```python
from build123d import *

# Parameters (mm, degrees)
SKETCH006_R             = 1.75
SKETCH006_W             = 6.5
SKETCH006_H             = 3
SKETCH006_W_2           = 11.5
PAD001_DEPTH            = 8.5
FILLET004_R             = 1
FILLET005_R             = 0.8
FILLET006_R             = 0.5
SKETCH007_W             = 25.7
SKETCH007_H             = 13
POCKET002_DEPTH         = 3
FILLET007_R             = 0.5
SKETCH008_R             = 1.8
POCKET003_DEPTH         = 2
BODY001_PLACEMENT_ANGLE = 180


with BuildPart() as part:
    # Sketch006 → Pad001 (new body)
    with BuildSketch(Plane.XZ):
        with BuildLine():
            Line((15.7, 8.35), (15.7, -0.06))
            Line((15.7, -0.06), (16.99, -0.06))
            ThreePointArc((18.99, -2.06), (18.404214, -0.645786), (16.99, -0.06))
            Line((18.99, -2.06), (18.99, -5.56))
            ThreePointArc((16.99, -7.56), (18.404214, -6.974214), (18.99, -5.56))
            Line((16.99, -7.56), (15.7, -7.56))
            Line((15.7, -8.35), (15.7, -7.56))
            ThreePointArc((14.7, -9.35), (15.407107, -9.057107), (15.7, -8.35))
            Line((14.7, -9.35), (12, -9.35))
            Line((12, -7.41), (12, -9.35))
            Line((-12, -7.41), (12, -7.41))
            Line((-12, -7.41), (-12, -9.35))
            Line((-12, -9.35), (-13.7, -9.35))
            ThreePointArc((-14.7, -8.35), (-14.407107, -9.057107), (-13.7, -9.35))
            Line((-14.7, -8.35), (-14.7, 10.64))
            ThreePointArc((-12.7, 12.64), (-14.114214, 12.054214), (-14.7, 10.64))
            Line((-12.7, 12.64), (-8.41, 12.64))
            ThreePointArc((-6.41, 10.64), (-6.995786, 12.054214), (-8.41, 12.64))
            Line((-6.41, 10.64), (-6.41, 9.35))
            Line((-6.41, 9.35), (14.7, 9.35))
            ThreePointArc((15.7, 8.35), (15.407107, 9.057107), (14.7, 9.35))
        make_face()
        with Locations((-10.16, 8.89)):
            Circle(SKETCH006_R, mode=Mode.SUBTRACT)
        with Locations((15.24, -3.81)):
            Circle(SKETCH006_R, mode=Mode.SUBTRACT)
        with Locations((-8.91, -3.81)):
            Rectangle(SKETCH006_W, SKETCH006_H, mode=Mode.SUBTRACT)
        with Locations((6.41, -3.81)):
            Rectangle(SKETCH006_W_2, SKETCH006_H, mode=Mode.SUBTRACT)
    extrude(amount=-PAD001_DEPTH)

    # Fillet004
    fillet004_edges = [part.edges().sort_by_distance(p)[0] for p in [
        (12.16, 4.25, -2.31),
        (0.66, 4.25, -2.31),
        (-12.16, 4.25, -2.31),
        (-5.66, 4.25, -2.31),
        (12.16, 4.25, -5.31),
        (-5.66, 4.25, -5.31),
        (-12.16, 4.25, -5.31),
        (0.66, 4.25, -5.31),
    ]]
    fillet(fillet004_edges, radius=FILLET004_R)

    # Fillet005
    fillet005_edges = [part.edges().sort_by_distance(p)[0] for p in [
        (15.7, 4.25, -7.56),
        (15.7, 4.25, -0.06),
        (-6.41, 4.25, 9.35),
        (12, 4.25, -9.35),
        (-12, 4.25, -9.35),
    ]]
    fillet(fillet005_edges, radius=FILLET005_R)

    # Fillet006
    fillet006_edges = [part.edges().sort_by_distance(p)[0] for p in [
        (-12, 4.25, -7.41),
        (12, 4.25, -7.41),
    ]]
    fillet(fillet006_edges, radius=FILLET006_R)

    # Sketch007 (on Face47 of Fillet006) → Pocket002 (cut)
    with BuildSketch(Plane(origin=(0, 8.5, 0), x_dir=(1, 0, 0), z_dir=(0, 1, 0))):
        Rectangle(SKETCH007_W, SKETCH007_H)
    extrude(amount=-POCKET002_DEPTH, mode=Mode.SUBTRACT)

    # Fillet007
    fillet007_edges = [part.edges().sort_by_distance(p)[0] for p in [
        (12.85, 7, 6.5),
        (12.85, 7, -6.5),
        (-12.85, 7, 6.5),
        (-12.85, 7, -6.5),
    ]]
    fillet(fillet007_edges, radius=FILLET007_R)

    # Sketch008 (on Face39 of Fillet007) → Pocket003 (cut)
    with BuildSketch(Plane(origin=(0, 5.5, 0), x_dir=(1, 0, 0), z_dir=(0, 1, 0))):
        Circle(SKETCH008_R)
        with BuildLine():
            Line((1.5, -6.5), (12.35, -6.5))
            ThreePointArc((12.35, -6.5), (12.703553, -6.353553), (12.85, -6))
            Line((12.85, -6), (12.85, -1.5))
            Line((12.85, -1.5), (3.5, -1.5))
            ThreePointArc((3.5, -1.5), (2.085786, -2.085786), (1.5, -3.5))
            Line((1.5, -3.5), (1.5, -6.5))
        make_face()
        with BuildLine():
            Line((-1.5, -6.5), (-12.35, -6.5))
            ThreePointArc((-12.85, -6), (-12.703553, -6.353553), (-12.35, -6.5))
            Line((-12.85, -6), (-12.85, -1.5))
            Line((-12.85, -1.5), (-3.5, -1.5))
            ThreePointArc((-1.5, -3.5), (-2.085786, -2.085786), (-3.5, -1.5))
            Line((-1.5, -3.5), (-1.5, -6.5))
        make_face()
        with BuildLine():
            Line((-1.5, 6.5), (-12.35, 6.5))
            ThreePointArc((-12.35, 6.5), (-12.703553, 6.353553), (-12.85, 6))
            Line((-12.85, 6), (-12.85, 1.5))
            Line((-12.85, 1.5), (-3.5, 1.5))
            ThreePointArc((-3.5, 1.5), (-2.085786, 2.085786), (-1.5, 3.5))
            Line((-1.5, 3.5), (-1.5, 6.5))
        make_face()
        with BuildLine():
            Line((1.5, 6.5), (12.35, 6.5))
            ThreePointArc((12.85, 6), (12.703553, 6.353553), (12.35, 6.5))
            Line((12.85, 6), (12.85, 1.5))
            Line((12.85, 1.5), (3.5, 1.5))
            ThreePointArc((1.5, 3.5), (2.085786, 2.085786), (3.5, 1.5))
            Line((1.5, 3.5), (1.5, 6.5))
        make_face()
    extrude(amount=-POCKET003_DEPTH, mode=Mode.SUBTRACT)


with BuildPart() as part_1:
    # Body001 placement: moved
    add(part.part.moved(Location((0, 8.5, 0))).rotate(Axis((0, 8.5, 0), (0, 0, 1)), BODY001_PLACEMENT_ANGLE))


solid = part_1.part
```
Here's how the part is built. I have some questions about the finished solid (model axes, mm). A direction names the side the tool comes from. Coordinates: 2 decimals unless noted, no trailing zeros. Write each loop counter-clockwise with the first axis right and the second up, starting at its lowest first coordinate (ties: lowest second). Pieces come first, ordered by that corner, then holes. Notation, with made-up numbers: M 50,6.25 L 60,6.25 A13 cw 60,13.25 Z; hole C 35.25,18 d11. An arc over 180 degrees is marked long. Answer as CSV lines item,"result". Start each with the question number.
Q1. Will these pins go through, and if not, where does the flat tip stop? pin 1 Ø5.5 at (x, z) = (8.5, -3) entering from -Y; pin 2 Ø1.8 at (x, y) = (9, 6) entering from -Z; pin 3 Ø1.5 at (x, z) = (-7, -3.5) entering from -Y; pin 4 Ø2 at (y, z) = (5, 9) entering from -X.
Q2. If we mould it in two halves opening along X, with no side actions, what happens to faces 4 (the flat face through (-18.99, 4, -4)), 5 (the cylindrical face through (14.415, 4.309, -9.049)), 6 (the flat face through (0, 2, 6.5))? For each: pulls with the +X half, pulls with the -X half, needs draft (parallel to the pull), parting line crosses it, or undercut.
Q3. Suppose I cut it at A-A, the plane x = 10.16. List the corners of the cut face in (y, z) for me.
Q4. Suppose I cut it at B-B, the plane x = -10.5. List the corners of the cut face in (y, z) for me.
Q5. For faces 1 (the cylindrical face through (-2.1, 3.99, 2.07)), 2 (the flat face through (-6, 7, -5.31)), 3 (the flat face through (-4, 4, 9.35)), which set-ups out of +Z, -Z, +X, -X, +Y, -Y let a thin tool reach every point of the face, with its end or its side?
Q6. Suppose I cut it at D-D, the plane y = 3.75. State how many separate pieces and enclosed holes the cut face has, then the cut area to 3 significant figures.
Q7. Suppose I cut it at C-C, the plane z = 8.89. List the corners of the cut face in (x, y) for me.
Q8. I need wall thicknesses on probe 1 along Z at (x, y) = (10, 1.5); probe 2 along Z at (x, y) = (10.16, 4.5); probe 3 along X at (y, z) = (2, 4.25). Which ranges of each line are inside material? Lowest first, please. Write a range as [from, to].
Entries:
1,pin 1,"stops at y = 3"
1,pin 2,"stops at z = -7.41"
1,pin 3,"passes through"
1,pin 4,"stops at x = -15.7"
2,face 4,"pulls with the -X half"
2,face 5,"pulls with the +X half"
2,face 6,"undercut"
3,outline,"M 0,-7.41 L 8.5,-7.41 L 8.5,-5.31 L 5,-5.31 L 5,-6.5 L 0,-6.5 Z; M 0,6.5 L 5,6.5 L 5,1.5 L 3,1.5 L 3,-1.5 L 5,-1.5 L 5,-2.31 L 8.5,-2.31 L 8.5,7.14 L 0,7.14 Z; M 0,10.64 L 8.5,10.64 L 8.5,12.64 L 0,12.64 Z"
4,outline,"M 0,-7.41 L 8.5,-7.41 L 8.5,-5.31 L 5,-5.31 L 5,-6.5 L 0,-6.5 Z; M 0,6.5 L 5,6.5 L 5,1.5 L 3,1.5 L 3,-1.5 L 5,-1.5 L 5,-2.31 L 8.5,-2.31 L 8.5,9.35 L 0,9.35 Z"
5,face 1,"-Y"
5,face 2,"+Y, -Y"
5,face 3,"+Z, -X, +Y, -Y"
6,separate pieces,"1"
6,enclosed holes,"7"
6,area,"315 mm²"
7,outline,"M -15.54,0 L 8.41,0 L 8.41,8.5 L -15.54,8.5 Z; M 11.91,0 L 14.7,0 L 14.7,8.5 L 11.91,8.5 Z"
8,probe 1,"z = [-7.41, -6.5], [6.5, 7.15], [10.63, 12.64]"
8,probe 2,"z = [-7.41, -6.5], [-1.5, 1.5], [6.5, 7.14], [10.64, 12.64]"
8,probe 3,"x = [-15.7, -12.85], [12.85, 14.7]"
